The listing builds one solid part. Answer for the finished solid, in the listing's coordinates (mm). A direction names the side the tool comes from. Give positions to 0.01 mm unless a question says otherwise; leave off trailing zeros. Order: outer loops, then holes, each group sorted by start corner. A loop starts at its lowest first (then second) coordinate and runs counter-clockwise, first axis right, second up. Notation, with made-up numbers: (68.5, 9) - (100.5, 9) arc R23 cw to (100.5, 48) - close; hole circle Ø4 at (-20, 6.25). An arc over 180 degrees is marked (long way). Answer as a JSON object with one key per item and string values. Group by question number.
Q1. Consider line 1 (Y direction, x = 0, z = 5); line 2 (X direction, y = -11, z = 7.5); line 3 (Z direction, x = 9, y = -10.5). Determine where each line is inside the solid, lowest interval first.
Q2. The mould has two halves that part along X. Classify faces 6 (the face through (-0.404, -41.926, 3.549)), 7 (the face through (-4.05, -36, 8)), 8 (the face through (5, -15, 8)), 9 (the face through (15, -30, 4)): released by +X, released by -X, zero draft, split by the parting line, or undercut.
Q3. For faces 1 (the face through (-10, -10.95, 8)), 2 (the face through (10, -19.05, 8)), 3 (the face through (4.05, -36, 8)), 4 (the face through (0, -50, 8)), 5 (the face through (-4.05, -55, 8)), determine the directions among +Z, -Z, +X, -X, +Y, -Y from which every point of the face is accessible in a straight line to the end or side of a thin tool.
Q4. A cutting plane is placed at D-D, the plane y = -8. Give the vertices of the cut face in (x, z).
Q5. A cutting plane is placed at B-B, the plane x = 0. Give the vertices of the cut face in (y, z).
Q6. Given pin 1 (1.6 mm diameter, centred on x = -8.5, z = 8, fed in from -Y); pin 2 (1.2 mm diameter, centred on x = 1.5, z = 8, fed in from +Y); pin 3 (4 mm diameter, centred on x = -1.5, y = -29, fed in from +Z), each flat-ended and moving along its own axis, determine where each tip first touches the part or whether it passes through.
Q7. A cutting plane is placed at C-C, the plane z = 3.25. Give the vertices of the cut face in (x, y), and give its area (3 significant figures).
Q8. A cutting plane is placed at A-A, the plane y = -45. Give the vertices of the cut face in (x, z), and give its area (3 significant figures).
from build123d import *

# Parameters (mm, degrees)
SKETCH_W      = 30
SKETCH_H      = 60
PAD_DEPTH     = 7
FILLET_R      = 2
CHAMFER_SIZE  = 2
SKETCH001_R   = 3.1
POCKET_DEPTH  = 7.001
SKETCH002_W   = 10
SKETCH002_H   = 8.1
SKETCH002_W_2 = 8.1
SKETCH002_H_2 = 10
SKETCH002_H_3 = 8
PAD001_DEPTH  = 1.5


with BuildPart() as part:
    # Sketch → Pad (new body)
    with BuildSketch(Plane.XY):
        with Locations((0, -30)):
            Rectangle(SKETCH_W, SKETCH_H)
    extrude(amount=PAD_DEPTH)

    # Fillet
    fillet_edges = [part.edges().sort_by_distance(p)[0] for p in [
        (15, -60, 3.5),
        (15, 0, 3.5),
        (-15, 0, 3.5),
        (-15, -60, 3.5),
    ]]
    fillet(fillet_edges, radius=FILLET_R)

    # Chamfer
    chamfer_edges = [part.edges().sort_by_distance(p)[0] for p in [
        (15, -30, 0),
        (0, -60, 0),
        (-15, -30, 0),
        (0, 0, 0),
    ]]
    chamfer(chamfer_edges, length=CHAMFER_SIZE)

    # Sketch001 (on Face4 of Chamfer) → Pocket (cut, through all)
    with BuildSketch(Plane.XY.offset(7)):
        with Locations((0, -15)):
            Circle(SKETCH001_R)
        with Locations((0, -45)):
            Circle(SKETCH001_R)
    extrude(amount=-POCKET_DEPTH, mode=Mode.SUBTRACT)

    # Sketch002 (on Face4 of Pocket) → Pad001 (join)
    with BuildSketch(Plane.XY.offset(7)):
        with Locations((-10, -15)):
            Rectangle(SKETCH002_W, SKETCH002_H)
        with Locations((10, -15)):
            Rectangle(SKETCH002_W, SKETCH002_H)
        with Locations((0, -55)):
            Rectangle(SKETCH002_W_2, SKETCH002_H_2)
        with Locations((0, -36)):
            Rectangle(SKETCH002_W_2, SKETCH002_H_3)
    extrude(amount=PAD001_DEPTH)


solid = part.part
Reply:
{
 "1": {"line 1": "y = -60 to -48.1, -41.9 to -18.1, -11.9 to 0", "line 2": "x = -15 to -5, 5 to 15", "line 3": "z = 0 to 7"},
 "2": {"face 6": "undercut", "face 7": "released by -X", "face 8": "undercut", "face 9": "released by +X"},
 "3": {"face 1": "+Z, +X, -X, +Y", "face 2": "+Z, +X, -X, -Y", "face 3": "+Z, +X, +Y, -Y", "face 4": "+Z, +X, -X", "face 5": "+Z, -X, +Y, -Y"},
 "4": {"outline": "(-15, 2) - (-13, 0) - (13, 0) - (15, 2) - (15, 7) - (-15, 7) - close"},
 "5": {"outline": "(-60, 2) - (-58, 0) - (-48.1, 0) - (-48.1, 7) - (-50, 7) - (-50, 8.5) - (-60, 8.5) - close; (-41.9, 0) - (-18.1, 0) - (-18.1, 7) - (-32, 7) - (-32, 8.5) - (-40, 8.5) - (-40, 7) - (-41.9, 7) - close; (-11.9, 0) - (-2, 0) - (0, 2) - (0, 7) - (-11.9, 7) - close"},
 "6": {"pin 1": "stops at y = -19.05", "pin 2": "stops at y = -32", "pin 3": "stops at z = 7"},
 "7": {"outline": "(-15, -58) arc R2 ccw to (-13, -60) - (13, -60) arc R2 ccw to (15, -58) - (15, -2) arc R2 ccw to (13, 0) - (-13, 0) arc R2 ccw to (-15, -2) - close; hole circle Ø6.2 at (0, -45); hole circle Ø6.2 at (0, -15)", "area": "1,740 mm^2"},
 "8": {"outline": "(-15, 2) - (-13, 0) - (-3.1, 0) - (-3.1, 7) - (-15, 7) - close; (3.1, 0) - (13, 0) - (15, 2) - (15, 7) - (3.1, 7) - close", "area": "163 mm^2"}
}
